from build123d import *

# Parameters (mm, degrees)
SKETCH1_R           = 10.16
BOSS_EXTRUDE1_DEPTH = 29.8958
SKETCH2_R           = 10.9728
BOSS_EXTRUDE2_DEPTH = 21.4122
SKETCH3_R           = 6.9342
BOSS_EXTRUDE3_DEPTH = 1.8288
BOSS_EXTRUDE4_START = -53.1368
SKETCH4_R           = 2.9718
BOSS_EXTRUDE4_DEPTH = 65.3542
CUT_EXTRUDE1_DEPTH  = 1.8288


with BuildPart() as part:
    # Sketch1 → Boss-Extrude1 (new body)
    with BuildSketch(Plane(origin=(0, 0, 0), x_dir=(1, 0, 0), z_dir=(0, 1, 0))):
        Circle(SKETCH1_R)
    extrude(amount=BOSS_EXTRUDE1_DEPTH)

    # Sketch2 → Boss-Extrude2 (add)
    with BuildSketch(Plane(origin=(0, 29.8958, 0), x_dir=(1, 0, 0), z_dir=(0, 1, 0))):
        Circle(SKETCH2_R)
    extrude(amount=BOSS_EXTRUDE2_DEPTH)

    # Sketch3 → Boss-Extrude3 (add)
    with BuildSketch(Plane(origin=(0, 51.308, 0), x_dir=(1, 0, 0), z_dir=(0, 1, 0))):
        Circle(SKETCH3_R)
    extrude(amount=BOSS_EXTRUDE3_DEPTH)

    # Sketch4 → Boss-Extrude4 (add)
    with BuildSketch(Plane(origin=(0, 53.1368, 0), x_dir=(1, 0, 0), z_dir=(0, 1, 0)).offset(BOSS_EXTRUDE4_START)):
        Circle(SKETCH4_R)
    extrude(amount=BOSS_EXTRUDE4_DEPTH)

    # Sketch5 → Cut-Extrude1 (cut)
    with BuildSketch(Plane(origin=(0, 53.1368, 0), x_dir=(1, 0, 0), z_dir=(0, 1, 0))):
        with BuildLine():
            Line((-3.529046421, 5.969), (3.529046421, 5.969))
            ThreePointArc((3.529046421, 5.969), (0, 6.9342), (-3.529046421, 5.969))
        make_face()
        with BuildLine():
            Line((3.529046421, -5.969), (-3.529046421, -5.969))
            ThreePointArc((-3.529046421, -5.969), (0, -6.9342), (3.529046421, -5.969))
        make_face()
    extrude(amount=-CUT_EXTRUDE1_DEPTH, mode=Mode.SUBTRACT)


solid = part.part
Geometry check sheet. Reference: the model listing, model coordinates, mm. A direction names the side the tool comes from. Give positions to 0.01 mm unless a question says otherwise; leave off trailing zeros. Write each loop counter-clockwise with the first axis right and the second up, starting at its lowest first coordinate (ties: lowest second). Pieces come first, ordered by that corner, then holes.
1) Set-up check for faces 1 (the face through (0, 52, -5.969)), 2 (the face through (-1.323, 14.739, -10.074)), 3 (the face through (2.835, 59.16, -0.893)), 4 (the face through (0, 52, 5.969)): record each of +Z, -Z, +X, -X, +Y, -Y from which the full face is reachable in a straight line by a thin tool's end or side.
Values follow:
face 1: -Z, +X, -X, +Y
face 2: -Y
face 3: +Y
face 4: +Z, +X, -X, +Y
2) Cross-section at B-B (z = 0). Record the boundary of the cut face in (x, y).
Values follow:
outline: (-10.97, 29.9) - (-10.16, 29.9) - (-10.16, 0) - (10.16, 0) - (10.16, 29.9) - (10.97, 29.9) - (10.97, 51.31) - (6.93, 51.31) - (6.93, 53.14) - (2.97, 53.14) - (2.97, 65.35) - (-2.97, 65.35) - (-2.97, 53.14) - (-6.93, 53.14) - (-6.93, 51.31) - (-10.97, 51.31) - close
3) Cross-section at C-C (y = 54). Record the boundary of the cut face in (x, z), plus the area to 3 significant figures.
Values follow:
outline: circle Ø5.94 at (0, 0)
area: 27.7 mm2
4) Cross-section at D-D (x = -9.25). Record the boundary of the cut face in (y, z).
Values follow:
outline: (0, -4.2) - (29.9, -4.2) - (29.9, -5.9) - (51.31, -5.9) - (51.31, 5.9) - (29.9, 5.9) - (29.9, 4.2) - (0, 4.2) - close
5) Go/stop test with flat-tipped pins: pin 1 Ø4 at (x, z) = (8.5, -6) entering from +Y; pin 2 Ø1.5 at (x, y) = (-8, 18) entering from +Z; pin 3 Ø1.5 at (x, y) = (0.5, 52.5) entering from -Z. Record where each tip stops, or that it passes through.
Values follow:
pin 1: stops at y = 51.31
pin 2: stops at z = 7.12
pin 3: stops at z = -5.97
6) Thickness scan on line 1 (Y direction, x = 5, z = 3.75); line 2 (X direction, y = 7, z = -0.25); line 3 (Z direction, x = 8.5, y = 38.5). Record the ranges inside material, lowest first.
Values follow:
line 1: y = 0 to 53.14
line 2: x = -10.16 to 10.16
line 3: z = -6.94 to 6.94
7) Cross-section at A-A (x = 0). Record the boundary of the cut face in (y, z), plus the area to 3 significant figures.
Values follow:
outline: (0, -10.16) - (29.9, -10.16) - (29.9, -10.97) - (51.31, -10.97) - (51.31, -5.97) - (53.14, -5.97) - (53.14, -2.97) - (65.35, -2.97) - (65.35, 2.97) - (53.14, 2.97) - (53.14, 5.97) - (51.31, 5.97) - (51.31, 10.97) - (29.9, 10.97) - (29.9, 10.16) - (0, 10.16) - close
area: 1,170 mm2
